Check sheet for the drawn part. Datum: minimum x, y, z corner. Units: mm. A direction names the side the tool comes from. Give positions to 0.01 mm unless a question says otherwise; leave off trailing zeros. Write each loop counter-clockwise with the first axis right and the second up, starting at its lowest first coordinate (ties: lowest second). Pieces come first, ordered by that corner, then holes. Notation, with made-up numbers: (-26.5, 5) -> (-5.5, 5) arc R16 ccw to (-5.5, 33) -> close; hole circle Ø3 at (-12, 85.25). An arc over 180 degrees is marked (long way). Answer as CSV lines item,"result". Start each with the question number.
1) Gauge pin test, flat ends, axial feed: pin 1 Ø3 at (y, z) = (1.5, 9) entering from +X; pin 2 Ø1 at (x, y) = (6.5, 7) entering from -Z; pin 3 Ø2 at (y, z) = (2.5, 30.5) entering from -X. Record the tip position at first contact, or that the pin passes through.
2) Tool access check on the marked faces 1 and 2. Record the directions out of +Z, -Z, +X, -X, +Y, -Y that give a thin tool (end or side, any length) a straight path to the whole face; none if there is none.
3) Sectioned sample at B-B on x = 4. Record the cut outline in (y, z).
4) Material ranges on L1, parallel to Z at x = 1.75, y = 7.25; L2, parallel to X at y = 4.5, z = 42.5; L3, parallel to Z at x = 3.25, y = 6, recorded low to high.
5) Sectioned sample at A-A on y = 4. Record the cut outline in (x, z).
6) Sectioned sample at C-C on z = 30.5. Record the cut outline in (x, y), and give its area (3 significant figures).
7) Sectioned sample at D-D on x = 0.5. Record the cut outline in (y, z).
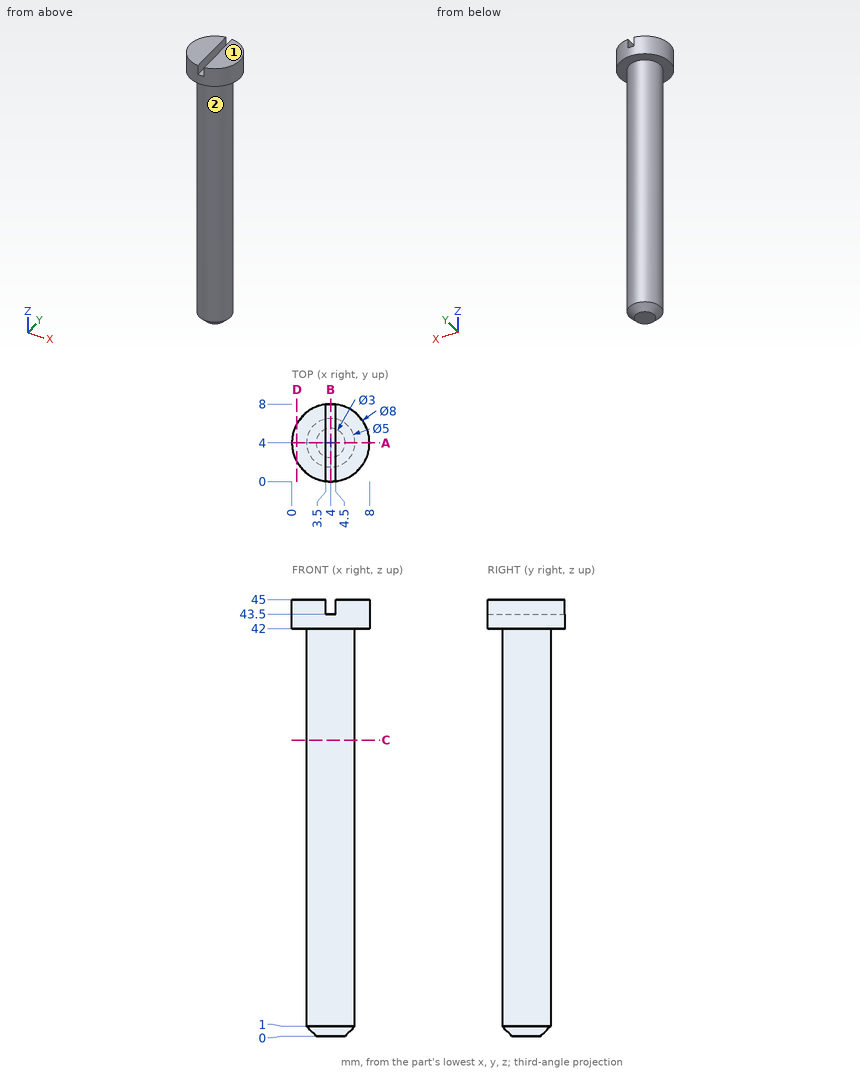
Ans:
1,pin 1,"stops at x = 6.29"
1,pin 2,"stops at z = 42"
1,pin 3,"stops at x = 1.55"
2,face 1,"+Z, +X, -X, +Y, -Y"
2,face 2,"-Z"
3,outline,"(0, 42) -> (1.5, 42) -> (1.5, 1) -> (2.5, 0) -> (5.5, 0) -> (6.5, 1) -> (6.5, 42) -> (8, 42) -> (8, 43.5) -> (0, 43.5) -> close"
4,L1,"z = 42 to 45"
4,L2,"x = 0.03 to 7.97"
4,L3,"z = 0.64 to 45"
5,outline,"(0, 42) -> (1.5, 42) -> (1.5, 1) -> (2.5, 0) -> (5.5, 0) -> (6.5, 1) -> (6.5, 42) -> (8, 42) -> (8, 45) -> (4.5, 45) -> (4.5, 43.5) -> (3.5, 43.5) -> (3.5, 45) -> (0, 45) -> close"
6,outline,"circle Ø5 at (4, 4)"
6,area,"19.6 mm²"
7,outline,"(2.06, 42) -> (5.94, 42) -> (5.94, 45) -> (2.06, 45) -> close"
